Autodesk Inventor part; units mm, degrees
ref_plane "YZ Plane" through (0, 0, 0) normal (1, 0, 0) x (0, 1, 0)
ref_plane "XZ Plane" through (0, 0, 0) normal (0, 1, 0) x (-1, 0, 0)
ref_plane "XY Plane" through (0, 0, 0) normal (0, 0, 1) x (1, 0, 0)
sketch "Sketch1" plane through (0, 0, 0) normal (0, 0, 1) x (1, 0, 0)
  line L0 (0, 0) -> (42.3, 0)
  line L1 (42.3, 0) -> (42.3, 42.3)
  line L2 (42.3, 42.3) -> (0, 42.3)
  line L3 (0, 42.3) -> (0, 0)
  line L4 (45.3, -3) -> (45.3, 45.3)
  line L5 (-3, 45.3) -> (-3, -3)
  line L6 (-6, -3) -> (45.3, -3)
  line L7 (-3, 45.3) -> (48.3, 45.3)
  circle A0 centre (48.3, 40.8) radius 2.5
  arc A1 (48.3, 36.3) -> (48.3, 45.3) centre (48.3, 40.8) ccw
  line L8 (45.3, 36.3) -> (48.3, 36.3)
  circle A2 centre (-6, 1.5) radius 2.5
  arc A3 (-6, 6) -> (-6, -3) centre (-6, 1.5) ccw
  line L9 (-3, 6) -> (-6, 6)
  point P0 (45.3, 42.3)
  point P1 (45.3, 0)
  point P2 (-3, 0)
  point P3 (-3, 42.3)
  dimension "d0" = 42.3
  dimension "d1" = 42.3
  dimension "d3" = 3
  dimension "d5" = 3
  dimension "d29" = 3
  dimension "d43" = 3
  dimension "d50" = 5
  dimension "d51" = 9
  dimension "d52" = 3
  dimension "d61" = 5
  dimension "d62" = 9
  dimension "d63" = 3
extrude "Extrusion7" add sketch "Sketch1" along normal blind 1
sketch "Sketch3" plane through (0, 0, 1) normal (0, 0, 1) x (1, 0, 0)
  line L0 (0, 0) -> (0, 42.3)
  line L1 (0, 42.3) -> (42.3, 42.3)
  line L2 (42.3, 42.3) -> (42.3, 0)
  line L3 (42.3, 0) -> (0, 0)
  circle A0 centre (48.3, 40.8) radius 2.5
  circle A1 centre (-6, 1.5) radius 2.5
  line L4 (-3, 6) -> (-6, 6)
  arc A2 (-6, 6) -> (-6, -3) centre (-6, 1.5) ccw
  line L5 (-6, -3) -> (45.3, -3)
  line L6 (45.3, -3) -> (45.3, 36.3)
  line L7 (45.3, 36.3) -> (48.3, 36.3)
  arc A3 (48.3, 36.3) -> (48.3, 45.3) centre (48.3, 40.8) ccw
  line L8 (48.3, 45.3) -> (-3, 45.3)
  line L9 (-3, 45.3) -> (-3, 6)
  line L10 (0, 42.3) -> (0, 0)
  line L11 (-3, 24.15) -> (0, 24.15)
  line L12 (0, 24.15) -> (0, 18.15)
  line L13 (0, 18.15) -> (-3, 18.15)
  line L14 (-3, 18.15) -> (-3, 24.15)
  line L15 (42.3, 24.15) -> (45.3, 24.15)
  line L16 (45.3, 24.15) -> (45.3, 18.15)
  line L17 (45.3, 18.15) -> (42.3, 18.15)
  line L18 (42.3, 18.15) -> (42.3, 24.15)
  line L19 (18.15, 45.3) -> (24.15, 45.3)
  line L20 (24.15, 45.3) -> (24.15, 42.3)
  line L21 (24.15, 42.3) -> (18.15, 42.3)
  line L22 (18.15, 42.3) -> (18.15, 45.3)
  line L23 (42.3, 0) -> (0, 0)
  line L24 (18.15, 0) -> (24.15, 0)
  line L25 (24.15, 0) -> (24.15, -3)
  line L26 (24.15, -3) -> (18.15, -3)
  line L27 (18.15, -3) -> (18.15, 0)
  dimension "d66" = 6
  dimension "d67" = 6
  dimension "d68" = 6
  dimension "d69" = 6
  dimension "d70" = 18.15
  dimension "d71" = 18.15
  dimension "d72" = 18.15
extrude "Extrusion9" add sketch "Sketch3" along normal blind 10 contours L13 L9 L11 L0 | L3 L25 L5 L27 | L22 L8 L20 L1
properties part number "Stepper_Motor_Holder-SquareBar-Rev3"
Could you check a few things on this model? Use its own coordinates, in mm. A direction names the side the tool comes from. Give positions to 0.01 mm unless a question says otherwise; leave off trailing zeros. Order: outer loops, then holes, each group sorted by start corner. A loop starts at its lowest first (then second) coordinate and runs counter-clockwise, first axis right, second up. Notation, with made-up numbers: M 53,56 L 94,56 A16 ccw 94,69 Z; hole C 21,72 d7. An arc over 180 degrees is marked long. One line per question, with ' | ' between items.
1. I want a section at A-A (y = 31). List the corners of the cut face in (x, z) for me.
Results:
outline: M -3,0 L 0,0 L 0,1 L -3,1 Z; M 42.3,0 L 45.3,0 L 45.3,1 L 42.3,1 Z
2. I want a section at D-D (y = 1.5). List the corners of the cut face in (x, z) for me, and give its area (3 significant figures).
Results:
outline: M -10.5,0 L -8.5,0 L -8.5,1 L -10.5,1 Z; M -3.5,0 L 0,0 L 0,1 L -3.5,1 Z; M 42.3,0 L 45.3,0 L 45.3,1 L 42.3,1 Z | area: 8.50 mm²
3. For faces 1 (the face through (18.15, -2, 6)), 2 (the face through (-2, 24.15, 6)), 3 (the face through (-1, 18.15, 6)), which set-ups out of +Z, -Z, +X, -X, +Y, -Y let a thin tool reach every point of the face, with its end or its side?
Results:
face 1: +Z, -X, +Y, -Y | face 2: +Z, +X, -X, +Y | face 3: +Z, +X, -X, -Y
4. If I drill on line 1 (Y direction, x = 48.3, z = 0.7); line 2 (Y direction, x = -6, z = 0.2); line 3 (X direction, y = 22, z = 7.5), over which ranges is the centre line in solid material (lowest first)?
Results:
line 1: 36.3 to 38.3, 43.3 to 45.3 | line 2: -3 to -1, 4 to 6 | line 3: -3 to 0
5. I want a section at C-C (z = 6). List the corners of the cut face in (x, y) for me, and give its area (3 significant figures).
Results:
outline: M -3,18.15 L 0,18.15 L 0,24.15 L -3,24.15 Z; M 18.15,-3 L 24.15,-3 L 24.15,0 L 18.15,0 Z; M 18.15,42.3 L 24.15,42.3 L 24.15,45.3 L 18.15,45.3 Z | area: 54.0 mm²
6. I'm going to push flat-ended pins straight in: pin 1 (4 mm diameter, centred on y = 38.5, z = 4, fed in from -X); pin 2 (2.5 mm diameter, centred on y = 43.5, z = 6.5, fed in from +X); pin 3 (1.5 mm diameter, centred on x = -2, z = 5, fed in from +Y); pin 4 (0.9 mm diameter, centred on y = -1, z = 5.5, fed in from -X). Where does each tip first touch, or does it pass through?
Results:
pin 1: through | pin 2: x = 24.15 | pin 3: y = 24.15 | pin 4: x = 18.15
